from build123d import *

# Parameters (mm, degrees)
F0_W     = 50.8
F0_H     = 50.8
F1_DEPTH = 12.7
F2_W     = 6.35
F2_H     = 12.7
F2_H_2   = 10.934927
F3_DEPTH = 12.7
F4_SIZE  = 5.08
F5_R     = 22.225
F6_DEPTH = 6.35
F7_W     = 38.1
F7_H     = 44.45
F8_DEPTH = 6.35


with BuildPart() as f1:
    # F0 (on Top) → F1 (new body)
    with BuildSketch(Plane.XY):
        with Locations((0.767379, -0.027555)):
            Rectangle(F0_W, F0_H)
    extrude(amount=-F1_DEPTH)

    # F2 (on face) → F3 (join)
    with BuildSketch(Plane(origin=(0, 0, -12.7), x_dir=(1, 0, 0), z_dir=(0, 0, -1))):
        with Locations((-21.457621, 19.077555)):
            Rectangle(F2_W, F2_H)
        with Locations((22.992379, 19.077555)):
            Rectangle(F2_W, F2_H)
        with Locations((-21.457621, -19.022445)):
            Rectangle(F2_W, F2_H)
        with Locations((22.992379, -19.904981)):
            Rectangle(F2_W, F2_H_2)
    extrude(amount=F3_DEPTH)

    # F4
    f4_edges = [f1.edges().sort_by_distance(p)[0] for p in [
        (-21.457621, -12.727555, -25.4),
        (-18.282621, -19.077555, -25.4),
        (19.817379, -19.077555, -25.4),
        (22.992379, -12.727555, -25.4),
        (-18.282621, 19.022445, -25.4),
        (-21.457621, 12.672445, -25.4),
        (22.992379, 14.437518, -25.4),
        (19.817379, 19.904981, -25.4),
    ]]
    chamfer(f4_edges, length=F4_SIZE)

    # F5 (on face) → F6 (join)
    with BuildSketch(Plane.XY):
        Circle(F5_R)
    extrude(amount=F6_DEPTH)

    # F7 (on face) → F8 (join)
    with BuildSketch(Plane.XY):
        with Locations((-19.05, 0)):
            Rectangle(F7_W, F7_H)
    extrude(amount=F8_DEPTH)


solid = f1.part
Geometry: final body of the model. Coordinates: model frame, mm. A direction names the side the tool comes from. Coordinates: 2 decimals unless noted, no trailing zeros. Order: outer loops, then holes, each group sorted by start corner. A loop starts at its lowest first (then second) coordinate and runs counter-clockwise, first axis right, second up. Notation, with made-up numbers: M -29,78.5 L -8,78.5 A28 ccw -8,107.5 Z; hole C -35,88.25 d5. An arc over 180 degrees is marked long. One line per question, with ' | ' between items. Start each with the question number.
Item 1: Cut plane B-B, the plane z = -23. Return the cut outline in (x, y).
Item 2: Cut plane D-D, the plane z = -6.5. Return the cut outline in (x, y), then the cut area to 3 significant figures.
Item 3: Ray query, probe 1 along Y at (x, z) = (-19, -17); probe 2 along Y at (x, z) = (-13, 2) (3 decimals); probe 3 along Z at (x, y) = (19.5, -16.5). Return the intervals inside material, ascending. Write a range as [from, to].
Item 4: Pin query (flat end, axial travel): pin 1 Ø1.9 at (x, z) = (-11, 4) entering from -Y (3 decimals); pin 2 Ø3 at (x, y) = (-10, 5) entering from -Z; pin 3 Ø3 at (x, z) = (-14, 4.5) entering from +Y (3 decimals). Return the tip coordinate at first contact, or that it passes through.
Item 5: Set-up query: faces 1 (the flat face through (-22, -12.728, -16)), 2 (the flat face through (-18.283, 19, -16)), 3 (the flat face through (-19, 22.225, 3)), 4 (the flat face through (-24.633, 0, -10)). Return all of +Z, -Z, +X, -X, +Y, -Y with unobstructed straight access to the full face (end or side cutting, diameter ignored); none if empty.
Item 6: Cut plane C-C, the plane x = -20. Return the cut outline in (y, z) (3 decimals).
Item 7: Draft query along Y for faces 5 (the flat face through (0, 0, -12.7)), 6 (the cylindrical face through (22.22, -0.49, 3.13)), 7 (the flat face through (0, -25.428, -10)), 8 (the flat face through (-20.86, 20.52, -22.9)). Return one class per face: released by +Y, released by -Y, zero draft, split by the parting line, or undercut.
Item 8: Cut plane A-A, the plane y = 0. Return the cut outline in (x, z) (3 decimals), then the cut area to 3 significant figures.
A:
1) outline: M -24.63,-25.43 L -20.96,-25.43 L -20.96,-15.41 L -24.63,-15.41 Z; M -24.63,15.35 L -20.96,15.35 L -20.96,25.37 L -24.63,25.37 Z; M 22.5,-25.43 L 26.17,-25.43 L 26.17,-15.41 L 22.5,-15.41 Z; M 22.5,17.12 L 26.17,17.12 L 26.17,25.37 L 22.5,25.37 Z
2) outline: M -24.63,-25.43 L 26.17,-25.43 L 26.17,25.37 L -24.63,25.37 Z | area: 2,580 mm2
3) probe 1: y = [-25.43, -12.73], [12.67, 25.37] | probe 2: y = [-22.225, 22.225] | probe 3: z = [-12.7, 0]
4) pin 1: stops at y = -22.225 | pin 2: stops at z = -12.7 | pin 3: stops at y = 22.225
5) face 1: -Z, +X, -X | face 2: -Z, +Y, -Y | face 3: +Z, +X, -X, +Y | face 4: -Z, -X, +Y, -Y
6) outline: M -25.428,-22.037 L -14.445,-22.037 L -12.728,-20.32 L -12.728,-12.7 L 12.672,-12.7 L 12.672,-20.32 L 14.39,-22.037 L 25.372,-22.037 L 25.372,0 L 22.225,0 L 22.225,6.35 L -22.225,6.35 L -22.225,0 L -25.428,0 Z
7) face 5: undercut | face 6: split by the parting line | face 7: released by -Y | face 8: zero draft
8) outline: M -38.1,0 L -24.633,0 L -24.633,-12.7 L 26.167,-12.7 L 26.167,0 L 22.225,0 L 22.225,6.35 L -38.1,6.35 Z | area: 1,030 mm2
